Autodesk Inventor part; units mm, degrees
ref_plane "YZ Plane" through (0, 0, 0) normal (1, 0, 0) x (0, 1, 0)
ref_plane "XZ Plane" through (0, 0, 0) normal (0, 1, 0) x (-1, 0, 0)
ref_plane "XY Plane" through (0, 0, 0) normal (0, 0, 1) x (1, 0, 0)
sketch "Boceto1" plane through (0, 0, 0) normal (0, 0, 1) x (1, 0, 0)
  line L0 (0, 12.1119) -> (0, -11.4197) construction
  line L1 (-11.1817, 0) -> (11.1817, 0) construction
  line L2 (4.9434, 0.75) -> (5.5, 0.75)
  line L3 (4.9434, -0.75) -> (5.5, -0.75)
  line L4 (5.5, -0.75) -> (5.5, 0.75)
  line L5 (-0.75, 4.9434) -> (-0.75, 5.5)
  line L6 (0.75, 5.5) -> (-0.75, 5.5)
  line L7 (0.75, 4.9434) -> (0.75, 5.5)
  line L8 (-4.9434, -0.75) -> (-5.5, -0.75)
  line L9 (-5.5, 0.75) -> (-5.5, -0.75)
  line L10 (-4.9434, 0.75) -> (-5.5, 0.75)
  line L11 (0.75, -4.9434) -> (0.75, -5.5)
  line L12 (-0.75, -5.5) -> (0.75, -5.5)
  line L13 (-0.75, -4.9434) -> (-0.75, -5.5)
  arc A0 (-0.75, 4.9434) -> (-4.9434, 0.75) centre (0, 0) ccw
  arc A1 (-4.9434, -0.75) -> (-0.75, -4.9434) centre (0, 0) ccw
  arc A2 (0.75, -4.9434) -> (4.9434, -0.75) centre (0, 0) ccw
  arc A3 (4.9434, 0.75) -> (0.75, 4.9434) centre (0, 0) ccw
  circle A4 centre (0, 0) radius 5 construction
  point P0 (5.5, 0)
  dimension "d3" = 0.75
  dimension "d4" = 1.5
  dimension "d5" = 360
  dimension "d7" = 0.5
  dimension "d8" = 5
  dimension "d43" = 10
extrude "Extrusión1" add sketch "Boceto1" against normal blind 46
sketch "Boceto3" plane through (0, 0, -46) normal (0, 0, -1) x (-1, 0, 0)
  circle A0 centre (0, 0) radius 6.5
  dimension "d49" = 13
extrude "Extrusión3" add sketch "Boceto3" along normal blind 1
sketch "Boceto2" plane through (0, 0, -47) normal (0, 0, -1) x (-1, 0, 0)
  circle A0 centre (0, 0) radius 3.5
  dimension "d46" = 7
extrude "Extrusión2" cut sketch "Boceto2" against normal blind 40
properties part number "HIN-61 BISAGRA (BUJE PLASTICO)" material "Plástico ABS"
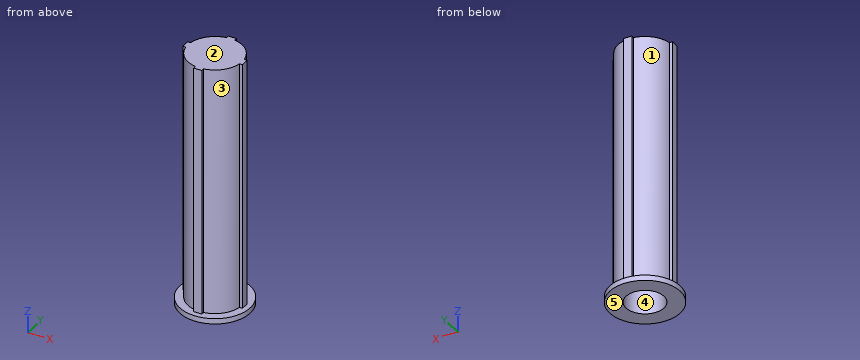
CAD build for the part. Positions are in the model's coordinates, mm. Face numbers are marked on the shaded views. A direction names the side the tool comes from. Round coordinates to 2 decimals unless told otherwise and drop trailing zeros. Order: outer loops, then holes, each group sorted by start corner. A loop starts at its lowest first (then second) coordinate and runs counter-clockwise, first axis right, second up. Notation, with made-up numbers: M -19,49.5 L 8,49.5 A30 cw 8,80.5 Z; hole C 23,53.25 d6. An arc over 180 degrees is marked long. Use one line per item in the form item = value.
Q1. Two-plate mould, pull along X, no slides. Class the marked faces 3, 4 and 5: +X half, -X half, draft (parallel to the pull), parting line (faces both ways), or undercut.
Recorded:
face_3 = +X half
face_4 = undercut
face_5 = draft
Q2. Saw through at D-D on x = -4.25. Give the cut face in (y, z), then the cut area to 3 significant figures.
Recorded:
outline = M -4.92,-47 L 4.92,-47 L 4.92,-46 L 2.63,-46 L 2.63,0 L -2.63,0 L -2.63,-46 L -4.92,-46 Z
area = 252 mm^2
Q3. Flat gauge pins, fed straight in: P1, Ø0.6, axis at x = 5.5, z = -24, coming from the -Y side; P2, Ø4, axis at y = -2.5, z = -26.5, coming from the +X side; P3, Ø2, axis at x = 4.5, z = -6.5, coming from the -Y side. Where does each tip first touch, or does it go through?
Recorded:
P1 = -0.75
P2 = 5.5
P3 = -3.57
Q4. Saw through at A-A on z = -30.5. Give the cut face in (x, y), then the cut area to 3 significant figures.
Recorded:
outline = M -5.5,-0.75 L -4.94,-0.75 A5 ccw -0.75,-4.94 L -0.75,-5.5 L 0.75,-5.5 L 0.75,-4.94 A5 ccw 4.94,-0.75 L 5.5,-0.75 L 5.5,0.75 L 4.94,0.75 A5 ccw 0.75,4.94 L 0.75,5.5 L -0.75,5.5 L -0.75,4.94 A5 ccw -4.94,0.75 L -5.5,0.75 Z; hole C 0,0 d7
area = 43.2 mm^2
Q5. Probe L1, parallel to Y at x = 0, z = -38.5; L2, parallel to Z at x = 0.5, y = -1; L3, parallel to X at y = 2.75, z = -29. List the from-to ranges inside material, lowest first.
Recorded:
L1 = -5.5 to -3.5, 3.5 to 5.5
L2 = -7 to 0
L3 = -4.18 to -2.17, 2.17 to 4.18
Q6. Which spindle directions (+Z, -Z, +X, -X, +Y, -Y) get a long thin tool onto all of the face, cutting with end or side? Do the marked faces 1 and 2. Say none if no direction does.
Recorded:
face_1 = +Z, -X, +Y
face_2 = +Z, +X, -X, +Y, -Y
Q7. Saw through at B-B on y = 0. Give the cut face in (x, z).
Recorded:
outline = M -6.5,-47 L -3.5,-47 L -3.5,-7 L 3.5,-7 L 3.5,-47 L 6.5,-47 L 6.5,-46 L 5.5,-46 L 5.5,0 L -5.5,0 L -5.5,-46 L -6.5,-46 Z
